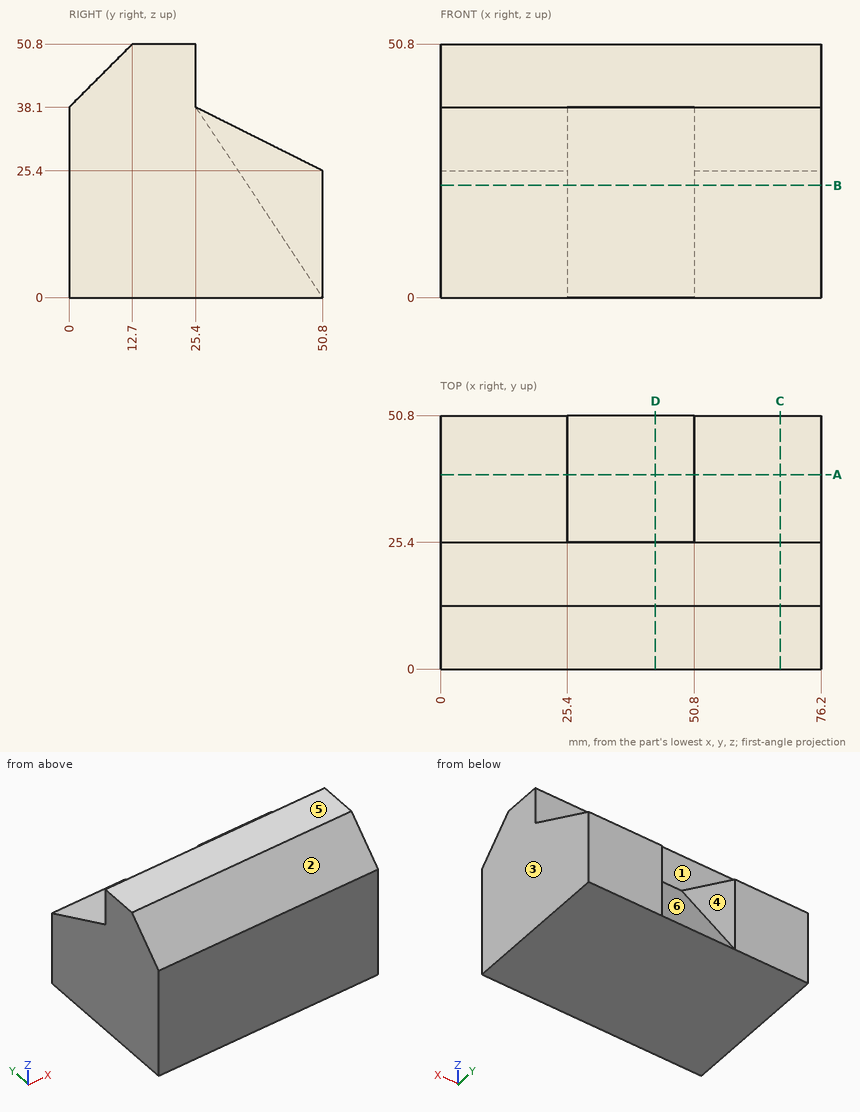
Geometry check sheet. Reference: drawing and pictorial views, mm from the part's lowest x, y, z. A direction names the side the tool comes from. Coordinates: 2 decimals unless noted, no trailing zeros. Write each loop counter-clockwise with the first axis right and the second up, starting at its lowest first coordinate (ties: lowest second). Pieces come first, ordered by that corner, then holes. Notation, with made-up numbers: (-10, -40) - (41, -40) arc R21 cw to (41, -27) - close; hole circle Ø5 at (80, -32). An arc over 180 degrees is marked (long way). Write item = value, one per line.
Q1. Access from +Z, -Z, +X, -X, +Y, -Y to the whole of each face (thin tool, end or side, straight path). Record for the marked faces 1 and 2.
Answer:
face_1 = +Z, +X, -X, +Y
face_2 = +Z, +X, -X, -Y
Q2. Cross-section at C-C (x = 68). Enter the section's corners in (y, z), plus the area to 3 significant figures.
Answer:
outline = (0, 0) - (50.8, 0) - (50.8, 25.4) - (25.4, 38.1) - (25.4, 50.8) - (12.7, 50.8) - (0, 38.1) - close
area = 2,020 mm²
Q3. Material ranges on L1, parallel to X at y = 46.5, z = 23.5; L2, parallel to Y at x = 33.5, z = 21; L3, parallel to Y at x = 66, z = 41, recorded low to high. Write a range as from..to.
Answer:
L1 = 0..25.4, 50.8..76.2
L2 = 0..36.8
L3 = 2.9..25.4
Q4. Cross-section at B-B (z = 22.5). Enter the section's corners in (x, y).
Answer:
outline = (0, 0) - (76.2, 0) - (76.2, 50.8) - (50.8, 50.8) - (50.8, 35.8) - (25.4, 35.8) - (25.4, 50.8) - (0, 50.8) - close
Q5. Cross-section at A-A (y = 39). Enter the section's corners in (x, z), plus the area to 3 significant figures.
Answer:
outline = (0, 0) - (76.2, 0) - (76.2, 31.3) - (50.8, 31.3) - (50.8, 17.7) - (25.4, 17.7) - (25.4, 31.3) - (0, 31.3) - close
area = 2,040 mm²
Q6. Mould release check, pull along X, two halves, no side actions. Record for the marked faces 3, 4, 5 and 6: released by +X, released by -X, zero draft, split by the parting line, or undercut.
Answer:
face_3 = released by +X
face_4 = undercut
face_5 = zero draft
face_6 = undercut
Q7. Cross-section at D-D (x = 43). Enter the section's corners in (y, z).
Answer:
outline = (0, 0) - (50.8, 0) - (25.4, 38.1) - (25.4, 50.8) - (12.7, 50.8) - (0, 38.1) - close
Q8. Go/stop test with flat-tipped pins: pin 1 Ø8 at (x, y) = (33.5, 39) entering from +Z; pin 2 Ø8 at (x, z) = (52.5, 42.5) entering from +Y; pin 3 Ø4 at (x, z) = (30, 12.5) entering from +Y. Record where each tip stops, or that it passes through.
Answer:
pin_1 = 23.7
pin_2 = 25.4
pin_3 = 43.8
